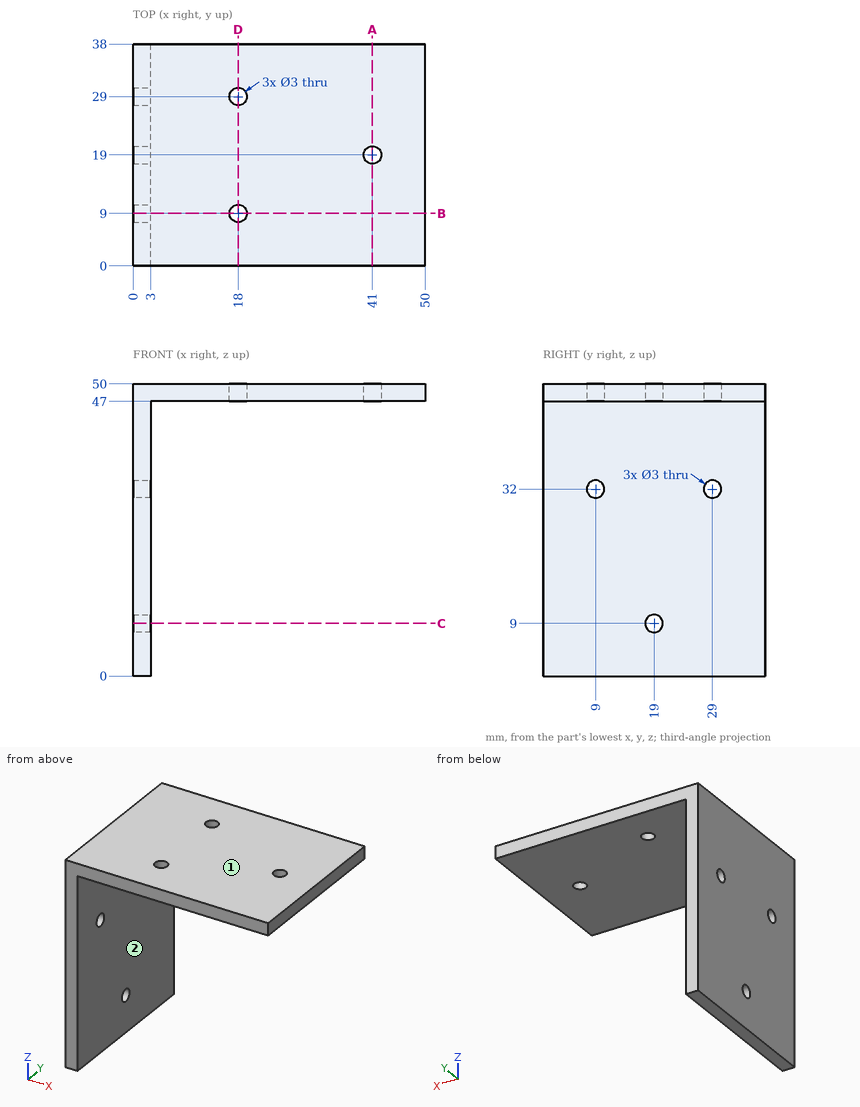
Print and shaded views of the part. All mm, measured from the part's lowest x, y and z. A direction names the side the tool comes from. Coordinates: 2 decimals unless noted, no trailing zeros. Write each loop counter-clockwise with the first axis right and the second up, starting at its lowest first coordinate (ties: lowest second). Pieces come first, ordered by that corner, then holes.
(1) Cut at C-C, the plane z = 9. List the corners of the cut face in (x, y), and give its area (3 significant figures).
(2) Cut at B-B, the plane y = 9. List the corners of the cut face in (x, z), and give its area (3 significant figures).
(3) Cut at D-D, the plane x = 18. List the corners of the cut face in (y, z), and give its area (3 significant figures).
(4) Flat gauge pins, fed straight in: pin 1 (1.8 mm diameter, centred on y = 29, z = 32, fed in from +X); pin 2 (12 mm diameter, centred on y = 5, z = 24, fed in from -X); pin 3 (4 mm diameter, centred on x = 18, y = 29, fed in from -Z); pin 4 (5 mm diameter, centred on y = 19, z = 9, fed in from +X). Where does each tip first touch, or does it go through?
(5) 3-axis set-ups, long thin cutter, end or side, ignore diameter. For the marked faces 1 and 2: which of +Z, -Z, +X, -X, +Y, -Y reach the whole face in a straight line?
(6) Cut at A-A, the plane x = 41. List the corners of the cut face in (y, z).
(7) Drill centre lines: probe 1 along Y at (x, z) = (18, 48.6); probe 2 along Y at (x, z) = (41, 47.95); probe 3 along Z at (x, y) = (14.5, 2). Where is each one in solid material? Low to high.
Geometry says:
1. outline: (0, 0) - (3, 0) - (3, 17.5) - (0, 17.5) - close; (0, 20.5) - (3, 20.5) - (3, 38) - (0, 38) - close
1. area: 105 mm2
2. outline: (0, 0) - (3, 0) - (3, 30.5) - (0, 30.5) - close; (0, 33.5) - (3, 33.5) - (3, 47) - (16.5, 47) - (16.5, 50) - (0, 50) - close; (19.5, 47) - (50, 47) - (50, 50) - (19.5, 50) - close
2. area: 273 mm2
3. outline: (0, 47) - (7.5, 47) - (7.5, 50) - (0, 50) - close; (10.5, 47) - (27.5, 47) - (27.5, 50) - (10.5, 50) - close; (30.5, 47) - (38, 47) - (38, 50) - (30.5, 50) - close
3. area: 96.0 mm2
4. pin 1: passes through
4. pin 2: stops at x = 0
4. pin 3: stops at z = 47
4. pin 4: stops at x = 3
5. face 1: +Z, +X, -X, +Y, -Y
5. face 2: -Z, +X, +Y, -Y
6. outline: (0, 47) - (17.5, 47) - (17.5, 50) - (0, 50) - close; (20.5, 47) - (38, 47) - (38, 50) - (20.5, 50) - close
7. probe 1: y = 0 to 7.5, 10.5 to 27.5, 30.5 to 38
7. probe 2: y = 0 to 17.5, 20.5 to 38
7. probe 3: z = 47 to 50
